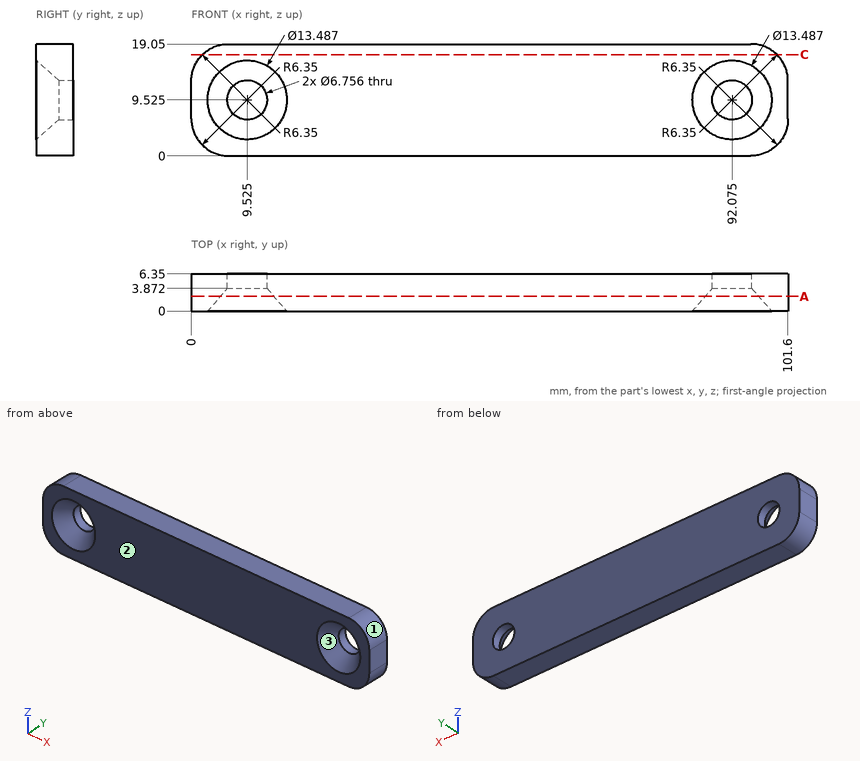
Answer from the drawing. Dimensions are ordinates in mm from the lowest x, y and z of the part. Give positions to 0.01 mm unless a question says otherwise; leave off trailing zeros. Loops run counter-clockwise (first coordinate to the right, second up) from the corner with the lowest first, then second, coordinate; pieces in that order, holes last. Notation, with made-up numbers: (-17.5, 77.5) -> (27.5, 77.5) arc R16 cw to (27.5, 100.5) -> close; hole circle Ø10 at (76, -14.75). An arc over 180 degrees is marked (long way). Answer as CSV lines item,"result".
Item 1: Consider line 1 (X direction, y = 5.25, z = 7); line 2 (X direction, y = 3, z = 7.5); line 3 (Z direction, x = 10.5, y = 5.5). Determine where each line is inside the solid, lowest interval first. Write a range as [from, to].
Returned:
line 1,"x = [0, 7.28], [11.77, 89.83], [94.32, 101.6]"
line 2,"x = [0, 5.92], [13.13, 88.47], [95.68, 101.6]"
line 3,"z = [0, 6.29], [12.76, 19.05]"
Item 2: Find section C-C on z = 17.25. Give the vertices of the cut face in (x, y), plus the area to 3 significant figures.
Returned:
outline,"(1.92, 0) -> (99.68, 0) -> (99.68, 6.35) -> (1.92, 6.35) -> close"
area,"621 mm²"
Item 3: Determine the mould class of the marked faces 1, 2 and 3 for opening direction X: +X half, -X half, draft (parallel to the pull), parting line (faces both ways), or undercut.
Returned:
face 1,"+X half"
face 2,"draft"
face 3,"undercut"
Item 4: Each of these flat-tipped pins is pushed along its axis until it touches: pin 1 (8 mm diameter, centred on x = 9.525, z = 9.525, fed in from -Y) (1 decimal); pin 2 (3 mm diameter, centred on y = 2, z = 6.5, fed in from -X). Where does it stop, or does it pass through?
Returned:
pin 1,"stops at y = 3.2"
pin 2,"stops at x = 0"
Item 5: Find section A-A on y = 2.5. State how many separate pieces and enclosed holes the cut face has, plus the area to 3 significant figures.
Returned:
separate pieces,"1"
enclosed holes,"2"
area,"1,770 mm²"
